```python
from build123d import *

# Parameters (mm, degrees)
F0_W     = 130
F0_H     = 50
F1_DEPTH = 2
F2_W     = 50
F2_H     = 50
F3_DEPTH = 60
F4_W     = 5
F4_H     = 5
F5_DEPTH = 70


with BuildPart() as f1:
    # F0 (on Top) → F1 (new body)
    with BuildSketch(Plane.XY):
        Rectangle(F0_W, F0_H)
    extrude(amount=F1_DEPTH)

    # F2 (on face) → F3 (join)
    with BuildSketch(Plane(origin=(0, 0, 0), x_dir=(1, 0, 0), z_dir=(0, 0, -1))):
        with Locations((40, 0)):
            Rectangle(F2_W, F2_H)
    extrude(amount=F3_DEPTH)

    # F4 (on face) → F5 (join)
    with BuildSketch(Plane(origin=(0, 0, 0), x_dir=(1, 0, 0), z_dir=(0, 0, -1))):
        with Locations((-62.5, 22.5)):
            Rectangle(F4_W, F4_H)
        with Locations((-62.5, -22.5)):
            Rectangle(F4_W, F4_H)
    extrude(amount=F5_DEPTH)


solid = f1.part
```
Design review of the part built by this model. Coordinates are the model's own, in mm. A direction names the side the tool comes from. Round coordinates to 2 decimals unless told otherwise and drop trailing zeros. Write each loop counter-clockwise with the first axis right and the second up, starting at its lowest first coordinate (ties: lowest second). Pieces come first, ordered by that corner, then holes. Notation, with made-up numbers: (34.25, -4.5) -> (75.25, -4.5) arc R8 cw to (75.25, 5.5) -> close; hole circle Ø9 at (24, 68). An arc over 180 degrees is marked (long way). Write item = value, one per line. Start each with the question number.
1) Take a section at B-B, the plane x = 49. State the section outline as (y, z) points, plus the area to 3 significant figures.
2) Take a section at A-A, the plane z = -4. State the section outline as (x, y) points, plus the area to 3 significant figures.
3) Wall thickness on probe 1 along X at (y, z) = (21, -57); probe 2 along Z at (x, y) = (-46.5, -15); probe 3 along Z at (x, y) = (17, 9.5): over which ranges is each line inside the solid? List them lowest first. Write a range as from..to.
4) Take a section at C-C, the plane y = 12. State the section outline as (x, z) points, plus the area to 3 significant figures.
5) Clearance check with flat-ended pins moving along their axes: pin 1 (15 mm diameter, centred on x = -5.5, y = 5, fed in from -Z); pin 2 (15 mm diameter, centred on x = 32.5, y = 0.5, fed in from -Z). State where each tip first meets the part, or that it passes through.
6) Tool access review of faces 1 (the face through (40, 0, -60)), 2 (the face through (29, 25, -28)), 3 (the face through (15, 0, -30)), 4 (the face through (-63, 20, -35)): name each direction out of +Z, -Z, +X, -X, +Y, -Y from which nothing blocks a thin tool from reaching the whole face with its end or side.
7) Take a section at D-D, the plane x = 2. State the section outline as (y, z) points, plus the area to 3 significant figures.
Results list:
q1.outline = (-25, -60) -> (25, -60) -> (25, 2) -> (-25, 2) -> close
q1.area = 3,100 mm²
q2.outline = (-65, -25) -> (-60, -25) -> (-60, -20) -> (-65, -20) -> close; (-65, 20) -> (-60, 20) -> (-60, 25) -> (-65, 25) -> close; (15, -25) -> (65, -25) -> (65, 25) -> (15, 25) -> close
q2.area = 2,550 mm²
q3.probe_1 = -65..-60, 15..65
q3.probe_2 = 0..2
q3.probe_3 = -60..2
q4.outline = (-65, 0) -> (15, 0) -> (15, -60) -> (65, -60) -> (65, 2) -> (-65, 2) -> close
q4.area = 3,260 mm²
q5.pin_1 = 0
q5.pin_2 = -60
q6.face_1 = -Z, +X, +Y, -Y
q6.face_2 = +Z, -Z, +X, -X, +Y
q6.face_3 = -Z, +Y, -Y
q6.face_4 = -Z, -X
q7.outline = (-25, 0) -> (25, 0) -> (25, 2) -> (-25, 2) -> close
q7.area = 100 mm²
